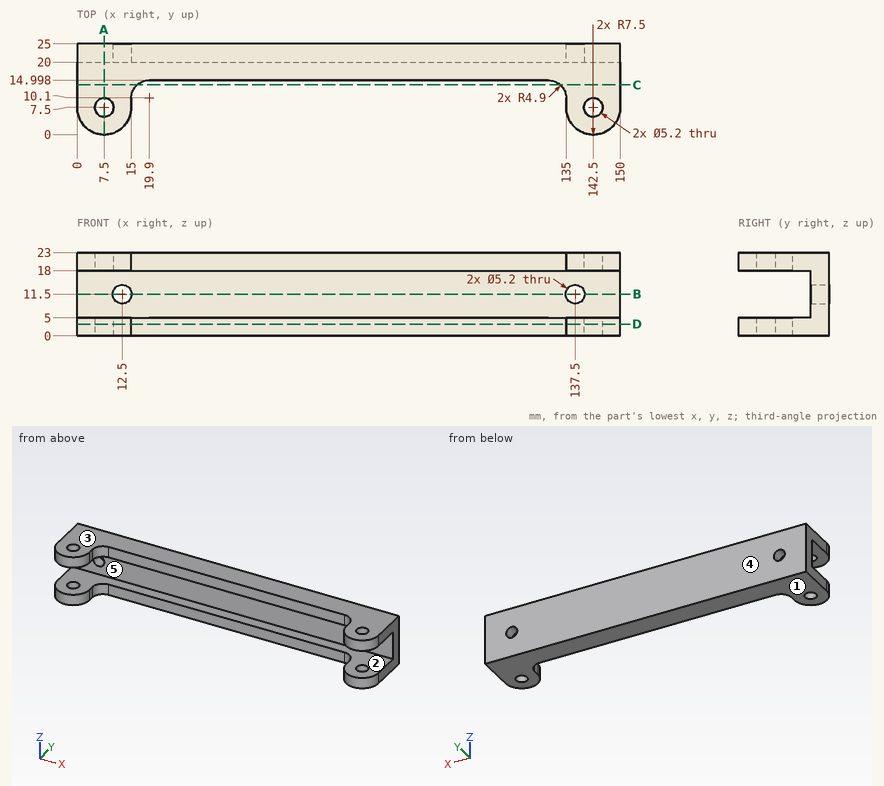
Can you work these out from the drawing? Everything is in mm from the part's minimum corner. A direction names the side the tool comes from. Round coordinates to 2 decimals unless told otherwise and drop trailing zeros. Order: outer loops, then holes, each group sorted by start corner. A loop starts at its lowest first (then second) coordinate and runs counter-clockwise, first axis right, second up. Notation, with made-up numbers: M 32,33.25 L 83,33.25 A9 cw 83,46.25 Z; hole C -36.5,-28 d3. An arc over 180 degrees is marked long. Answer as CSV lines item,"result".
Item 1: Imagine slicing it at A-A on x = 7.5. List the corners of the cut face in (y, z) for me.
From the geometry:
outline,"M 0,0 L 4.9,0 L 4.9,5 L 0,5 Z; M 0,18 L 4.9,18 L 4.9,23 L 0,23 Z; M 10.1,0 L 25,0 L 25,23 L 10.1,23 L 10.1,18 L 20,18 L 20,5 L 10.1,5 Z"
Item 2: For pin 1 (12 mm diameter, centred on x = 57, y = 8, fed in from -Z); pin 2 (2.5 mm diameter, centred on x = 53.5, z = 2.5, fed in from -Y), each with a flat end and sliding along its axis, tell me the tip position at first contact or that it passes through.
From the geometry:
pin 1,"through"
pin 2,"y = 15"
Item 3: Which directions (+Z, -Z, +X, -X, +Y, -Y) give clear straight access to the entire face, cutting with the end or side of a thin tool? Please do the marked faces 1 and 2.
From the geometry:
face 1,"-Z, +X, -X, +Y, -Y"
face 2,"+X, -X, -Y"
Item 4: Please list where these lines run through material, in increasing order: L1, parallel to X at y = 7.5, z = 20.6; L2, parallel to X at y = 22.5, z = 11.25; L3, parallel to Z at x = 83, y = 18. Write a range as [from, to].
From the geometry:
L1,"[0, 4.9], [10.1, 15], [135, 139.9], [145.1, 150]"
L2,"[0, 9.91], [15.09, 134.91], [140.09, 150]"
L3,"[0, 5], [18, 23]"
Item 5: Imagine slicing it at D-D on z = 3.25. List the corners of the cut face in (x, y) for me, and give its area (3 significant figures).
From the geometry:
outline,"M 0,7.5 A7.5 ccw 15,7.5 L 15,10.1 A4.9 cw 19.9,15 L 130.1,15 A4.9 cw 135,10.1 L 135,7.5 A7.5 ccw 150,7.5 L 150,25 L 0,25 Z; hole C 7.5,7.5 d5.2; hole C 142.5,7.5 d5.2"
area,"1,870 mm2"
Item 6: Imagine slicing it at B-B on z = 11.5. List the corners of the cut face in (x, y) for me.
From the geometry:
outline,"M 0,20 L 9.9,20 L 9.9,25 L 0,25 Z; M 15.1,20 L 134.9,20 L 134.9,25 L 15.1,25 Z; M 140.1,20 L 150,20 L 150,25 L 140.1,25 Z"
Item 7: We'd pull the mould along Z, two halves only. Please class the marked faces 3, 4 and 5: +Z half, -Z half, draft (parallel to the pull), parting line (faces both ways), or undercut.
From the geometry:
face 3,"+Z half"
face 4,"draft"
face 5,"undercut"
Item 8: Imagine slicing it at C-C on y = 13.75. List the corners of the cut face in (x, z) for me, and give its area (3 significant figures).
From the geometry:
outline,"M 0,0 L 16.63,0 L 16.63,5 L 0,5 Z; M 0,18 L 16.63,18 L 16.63,23 L 0,23 Z; M 133.37,0 L 150,0 L 150,5 L 133.37,5 Z; M 133.37,18 L 150,18 L 150,23 L 133.37,23 Z"
area,"333 mm2"
